Source: CAD feature listing. Evaluate the final solid. Frame: model axes, mm. Face numbers are marked on the shaded views. A direction names the side the tool comes from. Round coordinates to 2 decimals unless told otherwise and drop trailing zeros. Write each loop counter-clockwise with the first axis right and the second up, starting at its lowest first coordinate (ties: lowest second). Pieces come first, ordered by that corner, then holes.
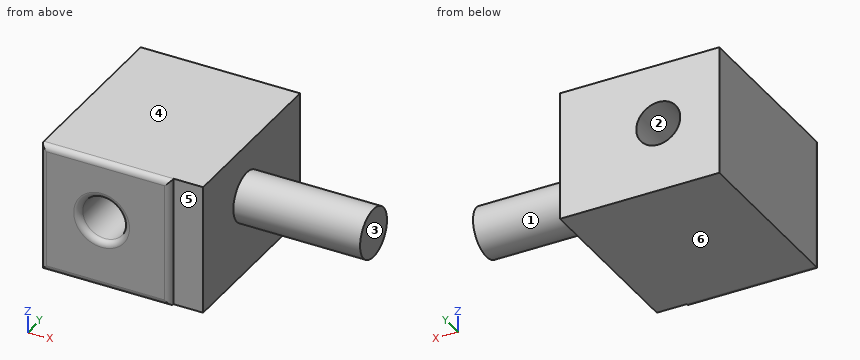
from build123d import *

# Parameters (mm, degrees)
F0_W     = 111.8744499981
F0_H     = 111.8744499981
F0_R     = 18.9654871471
F1_DEPTH = 157.988
F2_R     = 5.08
F3_DEPTH = 25.4
F4_R     = 21.242968454
F5_DEPTH = 109.22


with BuildPart() as f1:
    # F0 (on Front) → F1 (new body)
    with BuildSketch(Plane.XZ):
        with Locations((3.3725146204, -3.8376878947)):
            Rectangle(F0_W, F0_H)
        Circle(F0_R, mode=Mode.SUBTRACT)
    extrude(amount=F1_DEPTH)

    # F2
    f2_edges = [f1.edges().sort_by_distance(p)[0] for p in [
        (3.372515, -157.988, 52.099537),
        (-52.56471, -157.988, -3.837688),
        (3.372515, -157.988, -59.774913),
        (59.30974, -157.988, -3.837688),
        (-18.965487, -157.988, 0),
    ]]
    fillet(f2_edges, radius=F2_R)

    # F3 (add): a face of the model
    f3_faces = [f1.faces().sort_by_distance(p)[0] for p in [
        (59.3097396195, -76.454, -3.8376878947),
    ]]
    extrude(f3_faces, amount=F3_DEPTH)

    # F4 (on face) → F5 (join)
    with BuildSketch(Plane.YZ.offset(84.7097396195)):
        with Locations((-84.0359479189, 6.2909969129)):
            Circle(F4_R)
    extrude(amount=F5_DEPTH)


solid = f1.part
1) Section query B-B on z = 0. Return the cut outline in (x, y).
Taken from the geometry:
outline: (-52.56, -152.91) arc R5.08 ccw to (-47.48, -157.99) - (-24.05, -157.99) arc R5.08 ccw to (-18.97, -152.91) - (-18.97, 0) - (-52.56, 0) - close; (18.97, -152.91) arc R5.08 ccw to (24.05, -157.99) - (54.23, -157.99) arc R5.08 ccw to (59.31, -152.91) - (84.71, -152.91) - (84.71, -104.33) - (193.93, -104.33) - (193.93, -63.75) - (84.71, -63.75) - (84.71, 0) - (18.97, 0) - close
2) Pull-direction query (Z, two-part tool) for the marked faces 1, 2, 3 and 4; classes: released by +Z, released by -Z, zero draft, split by the parting line, or undercut.
Taken from the geometry:
face 1: split by the parting line
face 2: undercut
face 3: zero draft
face 4: released by +Z
3) Contact query for flat-ended pins moving along their axis: P1, Ø3, axis at y = -138.5, z = -46, coming from the +X side; P2, Ø20.5, axis at x = 75, z = -7, coming from the -Y side; P3, Ø1, axis at x = 97.5, y = -72.5, coming from the +Z side. Output: stop coordinate, or through.
Taken from the geometry:
P1: stops at x = 84.71
P2: stops at y = -152.91
P3: stops at z = 24.44
4) Section query A-A on x = 0. Return the cut outline in (y, z).
Taken from the geometry:
outline: (-157.99, -54.69) arc R5.08 ccw to (-152.91, -59.77) - (0, -59.77) - (0, -18.97) - (-152.91, -18.97) arc R5.08 ccw to (-157.99, -24.05) - close; (-157.99, 24.05) arc R5.08 ccw to (-152.91, 18.97) - (0, 18.97) - (0, 52.1) - (-152.91, 52.1) arc R5.08 ccw to (-157.99, 47.02) - close
5) Reachability of the marked faces 5 and 6 from +Z, -Z, +X, -X, +Y, -Y: full face, straight path, thin tool, end or side. Return the list, or none.
Taken from the geometry:
face 5: +Z, -Z, +X, -Y
face 6: -Z, +X, -X, +Y, -Y
6) Material intervals for line 1 (Z direction, x = 0, y = -101); line 2 (X direction, y = -13.5, z = 14); line 3 (X direction, y = -17.5, z = -7.5), sorted ascending.
Taken from the geometry:
line 1: z = -59.77 to -18.97, 18.97 to 52.1
line 2: x = -52.56 to -12.79, 12.79 to 84.71
line 3: x = -52.56 to -17.42, 17.42 to 84.71
7) Section query D-D on y = -121. Return the cut outline in (x, z).
Taken from the geometry:
outline: (-52.56, -59.77) - (84.71, -59.77) - (84.71, 52.1) - (-52.56, 52.1) - close; hole circle Ø37.93 at (0, 0)
8) Section query C-C on z = -42. Return the cut outline in (x, y), then the cut area to 3 significant figures.
Taken from the geometry:
outline: (-52.56, -152.91) arc R5.08 ccw to (-47.48, -157.99) - (54.23, -157.99) arc R5.08 ccw to (59.31, -152.91) - (84.71, -152.91) - (84.71, 0) - (-52.56, 0) - close
area: 21,500 mm2
